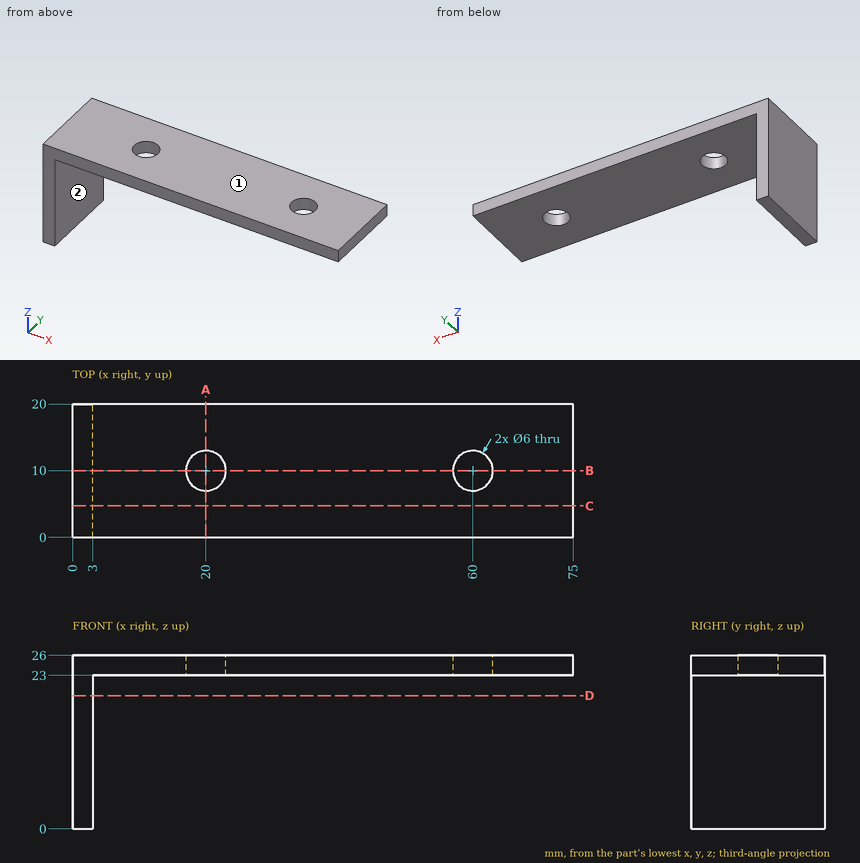
Can you work these out from the drawing? Everything is in mm from the part's minimum corner. A direction names the side the tool comes from. Give positions to 0.01 mm unless a question says otherwise; leave off trailing zeros. Order: outer loops, then holes, each group sorted by start corner. A loop starts at its lowest first (then second) coordinate and runs counter-clockwise, first axis right, second up. Notation, with made-up numbers: (83.25, 0) -> (116.25, 0) arc R15 cw to (116.25, 27) -> close; hole circle Ø9 at (86, 79.5). An arc over 180 degrees is marked (long way). Return JSON: item names as keys, results as strings.
1. For pin 1 Ø12 at (x, z) = (19, 12.5) entering from -Y; pin 2 Ø5 at (y, z) = (17, 19) entering from +X; pin 3 Ø8 at (y, z) = (12.5, 10.5) entering from -X; pin 4 Ø6 at (x, y) = (22, 6.5) entering from -Z, each with a flat end and sliding along its axis, tell me the tip position at first contact or that it passes through.
Answer list:
{"pin 1": "passes through", "pin 2": "stops at x = 3", "pin 3": "stops at x = 0", "pin 4": "stops at z = 23"}
2. Imagine slicing it at B-B on y = 10. List the corners of the cut face in (x, z) for me, then the cut area to 3 significant figures.
Answer list:
{"outline": "(0, 0) -> (3, 0) -> (3, 23) -> (17, 23) -> (17, 26) -> (0, 26) -> close; (23, 23) -> (57, 23) -> (57, 26) -> (23, 26) -> close; (63, 23) -> (75, 23) -> (75, 26) -> (63, 26) -> close", "area": "258 mm2"}
3. On a 3-axis mill with a long thin cutter (end or side, diameter ignored), from which of +Z, -Z, +X, -X, +Y, -Y can I reach the whole of each face in a straight line? I mean the marked faces 1 and 2. Say none if no direction works.
Answer list:
{"face 1": "+Z, +X, -X, +Y, -Y", "face 2": "-Z, +X, +Y, -Y"}
4. Imagine slicing it at C-C on y = 4.75. List the corners of the cut face in (x, z) for me, then the cut area to 3 significant figures.
Answer list:
{"outline": "(0, 0) -> (3, 0) -> (3, 23) -> (75, 23) -> (75, 26) -> (0, 26) -> close", "area": "294 mm2"}
5. I need wall thicknesses on line 1 (Y direction, x = 60, z = 24.15); line 2 (X direction, y = 2.25, z = 10); line 3 (Z direction, x = 32, y = 18.75). Which ranges of each line are inside material? Lowest first, please. Write a range as from..to.
Answer list:
{"line 1": "y = 0..7, 13..20", "line 2": "x = 0..3", "line 3": "z = 23..26"}
6. Imagine slicing it at D-D on z = 20. List the corners of the cut face in (x, y) for me, then the cut area to 3 significant figures.
Answer list:
{"outline": "(0, 0) -> (3, 0) -> (3, 20) -> (0, 20) -> close", "area": "60.0 mm2"}
7. Imagine slicing it at A-A on x = 20. List the corners of the cut face in (y, z) for me, then the cut area to 3 significant figures.
Answer list:
{"outline": "(0, 23) -> (7, 23) -> (7, 26) -> (0, 26) -> close; (13, 23) -> (20, 23) -> (20, 26) -> (13, 26) -> close", "area": "42.0 mm2"}
